from build123d import *

# Parameters (mm, degrees)
F0_R     = 14.28115
F0_R_2   = 2.5527
F1_DEPTH = 6.35


with BuildPart() as f1:
    # F0 (on Front) → F1 (new body)
    with BuildSketch(Plane.XZ):
        with BuildLine():
            Line((1289.421224, 766.672692), (-11.1125, 19.247415))
            ThreePointArc((-11.1125, 19.247415), (-19.28566, -11.134581), (11.1125, -19.247415))
            Line((11.1125, -19.247415), (1289.421229, 722.222692))
            Line((1289.421229, 722.222692), (1289.421224, 766.672692))
        make_face()
        Circle(F0_R, mode=Mode.SUBTRACT)
        with Locations((87.988181, 50.8)):
            Circle(F0_R_2, mode=Mode.SUBTRACT)
        Polygon((1670.421226, 766.672692), (1289.421224, 766.672692), (1289.421229, 722.222692), (1670.421226, 722.222692), align=None)
        with Locations((1302.121226, 744.447692)):
            Circle(F0_R_2, mode=Mode.SUBTRACT)
        with Locations((1327.521226, 744.447692)):
            Circle(F0_R_2, mode=Mode.SUBTRACT)
        with Locations((1352.921226, 744.447692)):
            Circle(F0_R_2, mode=Mode.SUBTRACT)
        with Locations((1378.321226, 744.447692)):
            Circle(F0_R_2, mode=Mode.SUBTRACT)
        with Locations((1403.721226, 744.447692)):
            Circle(F0_R_2, mode=Mode.SUBTRACT)
        with Locations((1429.121226, 744.447692)):
            Circle(F0_R_2, mode=Mode.SUBTRACT)
        with Locations((1454.521226, 744.447692)):
            Circle(F0_R_2, mode=Mode.SUBTRACT)
        with Locations((1479.921226, 744.447692)):
            Circle(F0_R_2, mode=Mode.SUBTRACT)
        with Locations((1505.321226, 744.447692)):
            Circle(F0_R_2, mode=Mode.SUBTRACT)
        with Locations((1530.721226, 744.447692)):
            Circle(F0_R_2, mode=Mode.SUBTRACT)
        with Locations((1556.121226, 744.447692)):
            Circle(F0_R_2, mode=Mode.SUBTRACT)
        with Locations((1581.521226, 744.447692)):
            Circle(F0_R_2, mode=Mode.SUBTRACT)
        with Locations((1606.921226, 744.447692)):
            Circle(F0_R_2, mode=Mode.SUBTRACT)
        with Locations((1632.321226, 744.447692)):
            Circle(F0_R_2, mode=Mode.SUBTRACT)
        with Locations((1657.721226, 744.447692)):
            Circle(F0_R_2, mode=Mode.SUBTRACT)
    extrude(amount=F1_DEPTH)


solid = f1.part
Input: part model. Units: mm. Frame: model coordinates. Give positions to 0.01 mm unless a question says otherwise; leave off trailing zeros. Write each loop counter-clockwise with the first axis right and the second up, starting at its lowest first coordinate (ties: lowest second). Pieces come first, ordered by that corner, then holes.
Q1. Section C-C, the plane x = 380. Output: boundary loops of the cut face in (y, z), plus the area to 3 significant figures.
Q2. Section B-B, the plane z = 477.5. Output: boundary loops of the cut face in (x, y).
Q3. Pull-direction query (X, two-part tool) for faces 1 (the face through (648.258, -3.131, 398.192)), 2 (the face through (-1.86, -3.13, 14.16)), 3 (the face through (641.32, -3.13, 346.3)), 4 (the face through (820, 0, 462)); classes: pulls with the +X half, pulls with the -X half, needs draft (parallel to the pull), parting line crosses it, or undercut.
Q4. First-contact query: P1, Ø4.5, axis at x = 1454.52, z = 744.45, coming from the +Y side; P2, Ø3, axis at x = 244.5, y = -1, coming from the +Z side; P3, Ø1.5, axis at y = -5, z = 150.5, coming from the -X side; P4, Ø1.5, axis at x = 1248, y = -1.5, coming from the +Z side. Flat tips, straight axial feed; report the tip coordinate or a pass-through.
Q5. Material intervals for probe 1 along Z at (x, y) = (0, -4.75); probe 2 along Z at (x, y) = (1308.5, -3.5); probe 3 along Z at (x, y) = (509, -3.25), sorted ascending.
Q6. Section A-A, the plane y = -4. State how many separate pieces and enclosed holes the cut face has, plus the area to 3 significant figures.
Filled in:
1. outline: (-6.35, 194.72) - (0, 194.72) - (0, 244.02) - (-6.35, 244.02) - close
1. area: 313 mm2
2. outline: (786.26, -6.35) - (867.51, -6.35) - (867.51, 0) - (786.26, 0) - close
3. face 1: pulls with the -X half
3. face 2: undercut
3. face 3: pulls with the +X half
3. face 4: needs draft
4. P1: passes through
4. P2: stops at z = 167.01
4. P3: stops at x = 215.96
4. P4: stops at z = 743.3
5. probe 1: z = -22.25 to -14.28, 14.28 to 25.63
5. probe 2: z = 722.22 to 766.67
5. probe 3: z = 269.55 to 318.16
6. separate pieces: 1
6. enclosed holes: 17
6. area: 78,500 mm2
